Check sheet for the modelled part. Datum: model origin and axes. Units: mm. A direction names the side the tool comes from. Round coordinates to 2 decimals unless told otherwise and drop trailing zeros. Write each loop counter-clockwise with the first axis right and the second up, starting at its lowest first coordinate (ties: lowest second). Pieces come first, ordered by that corner, then holes. Notation, with made-up numbers: (63.25, -19.75) -> (70.25, -19.75) arc R24 cw to (70.25, 5.25) -> close; hole circle Ø7 at (42, 46). An arc over 180 degrees is marked (long way). Use one line per item in the form item = value. Start each with the question number.
```python
from build123d import *

# Parameters (mm, degrees)
SKETCH2_W           = 24.86541407
SKETCH2_H           = 5.423229841
SKETCH2_H_2         = 4.001260317
CUT_EXTRUDE1_DEPTH  = 15
CIRPATTERN1_COUNT   = 2
CIRPATTERN1_ANGLE   = 90
CUT_EXTRUDE2_DEPTH  = 1.5
SKETCH4_R           = 5.5
BOSS_EXTRUDE1_DEPTH = 25
SKETCH5_R           = 1.5
BOSS_EXTRUDE2_DEPTH = 110


with BuildPart() as part:
    # Sketch1 → Revolve1 (revolve)
    with BuildSketch(Plane.XY, mode=Mode.PRIVATE) as revolve1_sk:
        with BuildLine():
            ThreePointArc((-74.569724464, 0), (-75.692690434, -7.615947487), (-77.869724464, -15))
            Line((-77.869724464, -15), (-72.619724464, -15))
            Line((-72.619724464, -15), (-66.369724464, -7.5))
            Line((-66.369724464, -7.5), (-56.369724464, -7.5))
            Line((-56.369724464, -7.5), (-55.889724464, -7.9))
            Line((-55.889724464, -7.9), (-50.139724464, -7.9))
            Line((-50.139724464, -7.9), (-49.659724464, -7.5))
            Line((-49.659724464, -7.5), (-44.659724464, -7.5))
            ThreePointArc((-44.659724464, -7.5), (-44.085344133, -8.375316627), (-43.245187811, -9))
            Line((-43.245187811, -9), (-40.559724464, -9))
            Line((-40.559724464, -9), (-34.259724464, -9))
            ThreePointArc((-34.259724464, -9), (-32.817493666, -8.603076001), (-31.746136172, -7.559154808))
            Line((-31.746136172, -7.559154808), (-31.746136172, -5))
            Line((-31.746136172, -5), (-30.246136172, -5))
            Line((-30.246136172, -5), (-30.246136172, -6))
            Line((-30.246136172, -6), (-28.746136172, -6))
            Line((-28.746136172, -6), (-28.746136172, -3.85))
            Line((-28.746136172, -3.85), (-25.083482145, -3.2))
            Line((-25.083482145, -3.2), (-25.083482145, 0))
            Line((-25.083482145, 0), (-74.569724464, 0))
        make_face()
    revolve(revolve1_sk.sketch.rotate(Axis((88.99, 0, 0), (-1, 0, 0)), 270), axis=Axis((88.99, 0, 0), (-1, 0, 0)))

    # Sketch2 → Cut-Extrude1 (cut)
    with BuildSketch(Plane(origin=(-31.746136172, 0, 0), x_dir=(0, 0, -1), z_dir=(1, 0, 0))):
        with Locations((0, -10.211614921)):
            Rectangle(SKETCH2_W, SKETCH2_H)
        with Locations((0, 9.500630158)):
            Rectangle(SKETCH2_W, SKETCH2_H_2)
    cut_extrude1 = extrude(amount=-CUT_EXTRUDE1_DEPTH, mode=Mode.SUBTRACT)

    # CirPattern1: Cut-Extrude1 ×2 about axis
    cirpattern1_axis = Axis((88.99, 0, 0), (-1, 0, 0))
    for i in range(1, CIRPATTERN1_COUNT):
        add(cut_extrude1.rotate(cirpattern1_axis, i * CIRPATTERN1_ANGLE / (CIRPATTERN1_COUNT - 1)), mode=Mode.SUBTRACT)

    # Sketch3 → Cut-Extrude2 (cut)
    with BuildSketch(Plane(origin=(-28.746136172, 0, 0), x_dir=(0, 0, -1), z_dir=(1, 0, 0))):
        with BuildLine():
            Line((2.75, -4.175823272), (2.75, -6.437196595))
            Line((2.75, -6.437196595), (5.963766818, -6.437196595))
            Line((5.963766818, -6.437196595), (6.43018781, 6.437196595))
            Line((6.43018781, 6.437196595), (2.75, 6.437196595))
            Line((2.75, 6.437196595), (2.75, 4.175823272))
            ThreePointArc((2.75, 4.175823272), (5, 0), (2.75, -4.175823272))
        make_face()
        with BuildLine():
            Line((-2.75, -6.437196595), (-2.75, -4.175823272))
            ThreePointArc((-2.75, -4.175823272), (-5, 0), (-2.75, 4.175823272))
            Line((-2.75, 4.175823272), (-2.75, 6.437196595))
            Line((-2.75, 6.437196595), (-6.280612264, 6.437196595))
            Line((-6.280612264, 6.437196595), (-6.280612264, -6.437196595))
            Line((-6.280612264, -6.437196595), (-2.75, -6.437196595))
        make_face()
    extrude(amount=-CUT_EXTRUDE2_DEPTH, mode=Mode.SUBTRACT)

    # Sketch4 → Boss-Extrude1 (add)
    with BuildSketch(Plane.XY.offset(7.5)):
        with Locations(Location((-38.752456137, 0, 0), (0, 0, 244.760598179))):
            Circle(SKETCH4_R)
    extrude(amount=BOSS_EXTRUDE1_DEPTH)

    # Sketch5 → Boss-Extrude2 (add)
    with BuildSketch(Plane(origin=(-25.083482145, 0, 0), x_dir=(0, 0, -1), z_dir=(1, 0, 0))):
        with Locations(Location((0, 0, 0), (0, 0, 180))):
            Circle(SKETCH5_R)
    extrude(amount=BOSS_EXTRUDE2_DEPTH)


solid = part.part
```
1. Depth check by flat-ended pin: pin 1 (1.3 mm diameter, centred on x = -30, y = -5, fed in from +Z); pin 2 (5 mm diameter, centred on x = -40, y = -1.5, fed in from -Z); pin 3 (1 mm diameter, centred on y = -5, z = 22.5, fed in from +X). Enter the tip coordinate at first touch or a pass-through.
2. Sectioned sample at A-A (z = 20). Enter the section's corners in (x, y), and give its area (3 significant figures).
3. Mould release check, pull along X, two halves, no side actions. Record for faces 1 (the face through (-66.67, -2.36, -7.5)), 2 (the face through (-28.746, -4, 0)), 3 (the face through (-33, 0, 7.5)): +X half, -X half, draft (parallel to the pull), parting line (faces both ways), or undercut.
4. Tool access check on faces 4 (the face through (-38, 7.5, 0)), 5 (the face through (-52.97, -5.34, 5.82)), 6 (the face through (-25.083, -1.5, -0.7)). Record the directions out of +Z, -Z, +X, -X, +Y, -Y that give a thin tool (end or side, any length) a straight path to the whole face; none if there is none.
5. Scan lines: probe 1 along Z at (x, y) = (-36, -1); probe 2 along X at (y, z) = (6, 6.5); probe 3 along X at (y, z) = (-6, -8). Record each from-to range of solid material in increasing order.
6. Sectioned sample at B-B (x = 69). Enter the section's corners in (y, z).
Returned:
q1.pin_1 = 2.75
q1.pin_2 = -7.5
q1.pin_3 = -35.59
q2.outline = circle Ø11 at (-38.75, 0)
q2.area = 95.0 mm^2
q3.face_1 = undercut
q3.face_2 = +X half
q3.face_3 = draft
q4.face_4 = +Z, -Z, +X, +Y
q4.face_5 = none
q4.face_6 = +X
q5.probe_1 = -7.5 to 32.5
q5.probe_2 = -75.98 to -67.49, -43.52 to -33.36
q5.probe_3 = -76.27 to -68.45
q6.outline = circle Ø3 at (0, 0)
